from build123d import *

# Parameters (mm, degrees)
F1_DEPTH = 3
F2_R     = 8.5
F3_DEPTH = 18
F4_SIZE  = 1.5


with BuildPart() as f1:
    # F0 (on Front) → F1 (new body)
    with BuildSketch(Plane.XZ):
        with BuildLine():
            Line((54.84, 12.7), (-54.84, 12.7))
            ThreePointArc((-54.84, 12.7), (-63.820256, 8.980256), (-67.54, 0))
            ThreePointArc((-67.54, 0), (-63.820256, -8.980256), (-54.84, -12.7))
            Line((-54.84, -12.7), (54.84, -12.7))
            ThreePointArc((54.84, -12.7), (63.820256, -8.980256), (67.54, 0))
            ThreePointArc((67.54, 0), (63.820256, 8.980256), (54.84, 12.7))
        make_face()
    extrude(amount=F1_DEPTH)

    # F2 (on face) → F3 (join)
    with BuildSketch(Plane.XZ.offset(3)):
        with Locations((-54.84, 0)):
            Circle(F2_R)
        with Locations((54.84, 0)):
            Circle(F2_R)
        with Locations((-18.28, 0)):
            Circle(F2_R)
        with Locations((18.28, 0)):
            Circle(F2_R)
    extrude(amount=F3_DEPTH)

    # F4
    f4_edges = [f1.edges().sort_by_distance(p)[0] for p in [
        (-63.34, -21, 0),
        (-26.78, -21, 0),
        (9.78, -21, 0),
        (46.34, -21, 0),
        (-26.78, -3, 0),
        (-63.34, -3, 0),
        (9.78, -3, 0),
        (46.34, -3, 0),
    ]]
    chamfer(f4_edges, length=F4_SIZE)


solid = f1.part
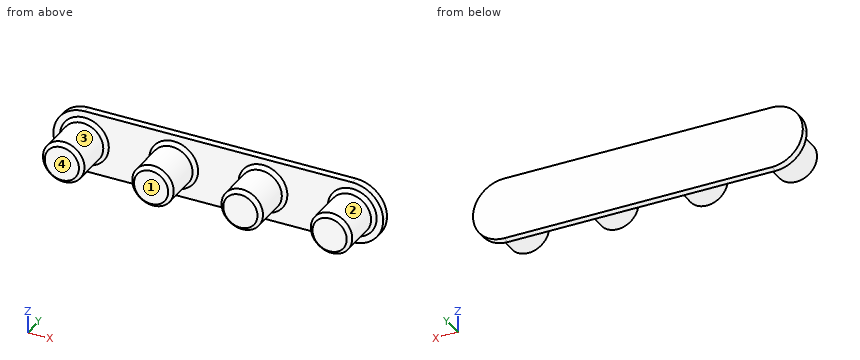
Design review of the part built by this model. Coordinates are the model's own, in mm. Face numbers are marked on the shaded views. A direction names the side the tool comes from. Round coordinates to 2 decimals unless told otherwise and drop trailing zeros. Write each loop counter-clockwise with the first axis right and the second up, starting at its lowest first coordinate (ties: lowest second). Pieces come first, ordered by that corner, then holes.
Item 1: Consider section A-A on y = -16. Give the boundary of the cut face in (x, z), and give its area (3 significant figures).
Item 2: For pin 1 Ø1.5 at (y, z) = (-17.5, 0.5) entering from +X; pin 2 Ø3 at (x, y) = (46, -11) entering from -Z; pin 3 Ø1 at (y, z) = (-15, -7) entering from -X; pin 4 Ø8 at (x, z) = (-2.5, -2) entering from +Y, all flat-tipped, find the tip position at first contact; note any pin that passes through.
Item 3: Consider section C-C on x = 0. Give the boundary of the cut face in (y, z), and give its area (3 significant figures).
Item 4: Wall thickness on L1, parallel to X at y = -14.5, z = 5; L2, parallel to X at y = -6.5, z = -0.25; L3, parallel to Y at x = -36.5, z = -4.75: over which ranges is each line inside the solid? List them lowest first.
Item 5: For the marked faces 1 and 2, list the 3-axis set-ups (+Z, -Z, +X, -X, +Y, -Y) from which the entire face can be reached by the end or side of a thin tool; tool diameter is ignored.
Item 6: Draft analysis for pull direction X (two halves, no side actions). For the marked faces 3 and 4, state which applies: released by +X, released by -X, zero draft, split by the parting line, or undercut.
Item 7: Consider section B-B on x = 18.28. Give the boundary of the cut face in (y, z), and give its area (3 significant figures).
Check values:
1. outline: circle Ø17 at (-54.84, 0); circle Ø17 at (-18.28, 0); circle Ø17 at (18.28, 0); circle Ø17 at (54.84, 0)
1. area: 908 mm2
2. pin 1: stops at x = 63.34
2. pin 2: stops at z = -4.29
2. pin 3: stops at x = -60.32
2. pin 4: stops at y = 0
3. outline: (-3, -12.7) - (0, -12.7) - (0, 12.7) - (-3, 12.7) - close
3. area: 76.2 mm2
4. L1: x = -61.71 to -47.97, -25.15 to -11.41, 11.41 to 25.15, 47.97 to 61.71
4. L2: x = -63.34 to -46.34, -26.78 to -9.78, 9.78 to 26.78, 46.34 to 63.34
4. L3: y = -3 to 0
5. face 1: +Z, -Z, +X, -X, -Y
5. face 2: -Y
6. face 3: undercut
6. face 4: zero draft
7. outline: (-21, -7) - (-19.5, -8.5) - (-4.5, -8.5) - (-3, -10) - (-3, -12.7) - (0, -12.7) - (0, 12.7) - (-3, 12.7) - (-3, 10) - (-4.5, 8.5) - (-19.5, 8.5) - (-21, 7) - close
7. area: 382 mm2
